Can you work these out from the drawing? Everything is in mm from the part's minimum corner. A direction names the side the tool comes from. Coordinates: 2 decimals unless noted, no trailing zeros. Order: outer loops, then holes, each group sorted by start corner. A loop starts at its lowest first (then second) coordinate and runs counter-clockwise, first axis right, second up. Notation, with made-up numbers: (-9, 11) - (32, 11) arc R22 ccw to (32, 47) - close; hole circle Ø9 at (51.25, 74.25). An arc over 180 degrees is marked (long way). Answer as CSV lines item,"result". Start each with the question number.
Q1. For the marked faces 5, 6, 7, 8 and 9, which set-ups out of +Z, -Z, +X, -X, +Y, -Y let a thin tool reach every point of the face, with its end or its side?
Q2. Suppose I cut it at B-B (y = 37.5). Please give me the cut outline in (x, z), then the cut area to 3 significant figures.
Q3. For pin 1 Ø7.5 at (x, y) = (6.5, 35) entering from +Z; pin 2 Ø13 at (y, z) = (19, 17) entering from -X; pin 3 Ø12 at (x, y) = (52.5, 30.5) entering from -Z; pin 4 Ø4 at (x, z) = (58.5, 2.5) entering from -Y, each with a flat end and sliding along its axis, tell me the tip position at first contact or that it passes through.
Q4. Suppose I cut it at A-A (x = 27.5). Please give me the cut outline in (y, z).
Q5. Thinking about a two-plate mould opening in Y: for the marked faces 1, 2, 3 and 4, which applies, released by +Y, released by -Y, zero draft, split by the parting line, or undercut?
Q6. I need wall thicknesses on line 1 (X direction, y = 31, z = 21); line 2 (Y direction, x = 58.4, z = 2.3); line 3 (Z direction, x = 44.5, y = 10.5). Which ranges of each line are inside material? Lowest first, please.
Q7. Suppose I cut it at C-C (z = 24). Please give me the cut outline in (x, y).
Q8. Suppose I cut it at D-D (y = 25.5). Please give me the cut outline in (x, z).
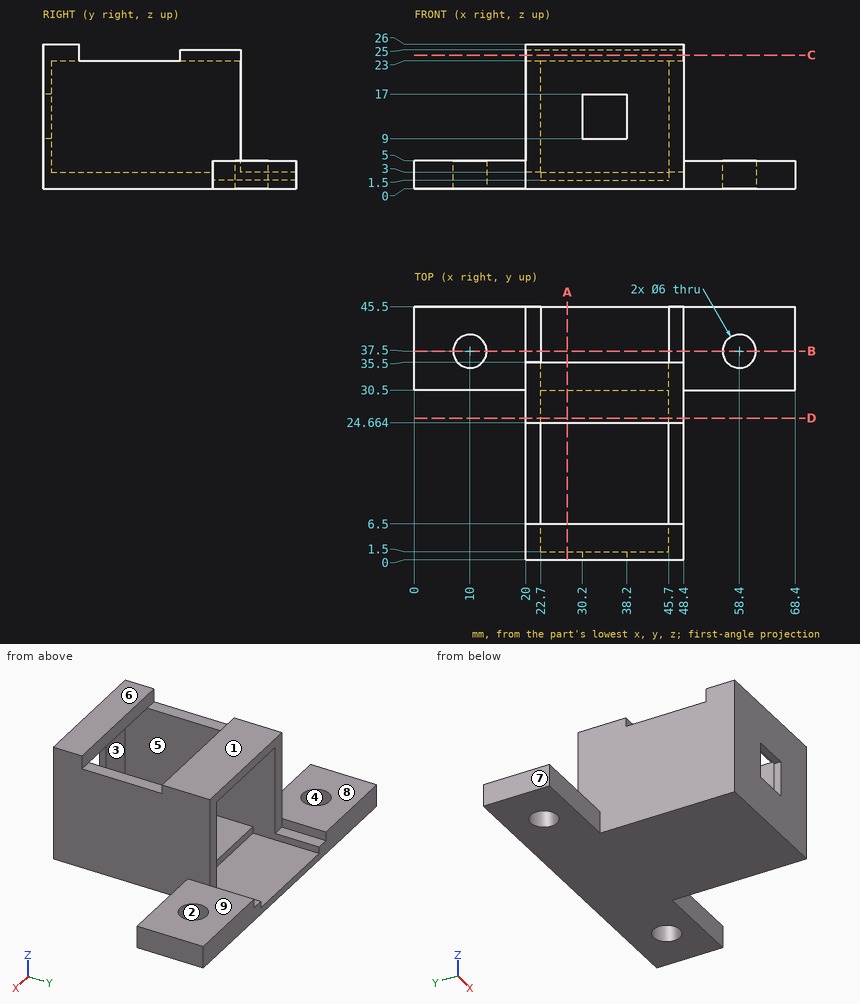
Here are the results:
1,face 5,"+Y"
1,face 6,"+Z, +X, -X, +Y, -Y"
1,face 7,"+Z, -Z, -X, +Y, -Y"
1,face 8,"+Z, -X, +Y, -Y"
1,face 9,"+Z, +X, +Y, -Y"
2,outline,"(0, 0) - (7, 0) - (7, 5) - (0, 5) - close; (13, 0) - (55.4, 0) - (55.4, 5) - (48.4, 5) - (48.4, 3) - (45.7, 3) - (45.7, 1.5) - (22.7, 1.5) - (22.7, 3) - (20, 3) - (20, 5) - (13, 5) - close; (61.4, 0) - (68.4, 0) - (68.4, 5) - (61.4, 5) - close"
2,area,"191 mm²"
3,pin 1,"stops at z = 5"
3,pin 2,"stops at x = 20"
3,pin 3,"stops at z = 0"
3,pin 4,"stops at y = 30.5"
4,outline,"(0, 0) - (45.5, 0) - (45.5, 1.5) - (30.5, 1.5) - (30.5, 3) - (1.5, 3) - (1.5, 23) - (6.5, 23) - (6.5, 26) - (0, 26) - close; (24.66, 23) - (35.5, 23) - (35.5, 25) - (24.66, 25) - close"
5,face 1,"zero draft"
5,face 2,"undercut"
5,face 3,"released by +Y"
5,face 4,"undercut"
6,line 1,"x = 20 to 22.7, 45.7 to 48.4"
6,line 2,"y = 30.5 to 34.5, 40.5 to 45.5"
6,line 3,"z = 0 to 3"
7,outline,"(20, 0) - (48.4, 0) - (48.4, 6.5) - (20, 6.5) - close; (20, 24.66) - (48.4, 24.66) - (48.4, 35.5) - (20, 35.5) - close"
8,outline,"(20, 0) - (48.4, 0) - (48.4, 25) - (20, 25) - close; hole (22.7, 3) - (45.7, 3) - (45.7, 23) - (22.7, 23) - close"
